The model under review builds one solid part; all positions refer to its coordinate system, in mm. A direction names the side the tool comes from. Round coordinates to 2 decimals unless told otherwise and drop trailing zeros. Loops run counter-clockwise (first coordinate to the right, second up) from the corner with the lowest first, then second, coordinate; pieces in that order, holes last. Notation, with made-up numbers: M 69.5,-17 L 89.5,-17 A28 ccw 89.5,10 Z; hole C -28,-16 d6. An arc over 180 degrees is marked long. One line per question, with ' | ' between items.
from build123d import *

# Parameters (mm, degrees)
CROQUIS1_W              = 40
CROQUIS1_H              = 41.5
CROQUIS1_R              = 2.5
SALIENTE_EXTRUIR1_DEPTH = 3
CROQUIS2_W              = 4
CROQUIS2_H              = 41.5
SALIENTE_EXTRUIR2_DEPTH = 45
CORTAR_EXTRUIR1_START   = 44
CROQUIS3_R              = 12.5
CROQUIS3_R_2            = 2.25
CORTAR_EXTRUIR1_DEPTH   = 4
SALIENTE_EXTRUIR4_START = 40
SALIENTE_EXTRUIR4_DEPTH = 4
CROQUIS6_W              = 40
CROQUIS6_H              = 9.5
CROQUIS6_H_2            = 9
SALIENTE_EXTRUIR5_DEPTH = 3
SALIENTE_EXTRUIR6_START = 46
CROQUIS7_W              = 40
CROQUIS7_H              = 61.549056497
CROQUIS7_R              = 2
SALIENTE_EXTRUIR6_DEPTH = 4


with BuildPart() as part:
    # Croquis1 → Saliente-Extruir1 (new body)
    with BuildSketch(Plane(origin=(0, 0, 0), x_dir=(1, 0, 0), z_dir=(0, 1, 0))):
        with Locations((20, -0.25)):
            Rectangle(CROQUIS1_W, CROQUIS1_H)
        with Locations((33.75, 14.25)):
            Circle(CROQUIS1_R, mode=Mode.SUBTRACT)
        with Locations((33.75, -14.75)):
            Circle(CROQUIS1_R, mode=Mode.SUBTRACT)
    extrude(amount=SALIENTE_EXTRUIR1_DEPTH)

    # Croquis2 → Saliente-Extruir2 (add)
    with BuildSketch(Plane(origin=(0, 0, 0), x_dir=(1, 0, 0), z_dir=(0, 1, 0))):
        with Locations((42, -0.25)):
            Rectangle(CROQUIS2_W, CROQUIS2_H)
    extrude(amount=SALIENTE_EXTRUIR2_DEPTH)

    # Croquis3 → Cortar-Extruir1 (cut)
    with BuildSketch(Plane(origin=(0, 0, 0), x_dir=(0, 0, -1), z_dir=(1, 0, 0)).offset(CORTAR_EXTRUIR1_START)):
        with Locations((-0.25, 24)):
            Circle(CROQUIS3_R)
        with Locations((15, 40)):
            Circle(CROQUIS3_R_2)
        with Locations((-15.5, 40)):
            Circle(CROQUIS3_R_2)
        with Locations((-15.5, 8)):
            Circle(CROQUIS3_R_2)
        with Locations((15, 8)):
            Circle(CROQUIS3_R_2)
    extrude(amount=-CORTAR_EXTRUIR1_DEPTH, mode=Mode.SUBTRACT)

    # Croquis5 → Saliente-Extruir4 (add)
    with BuildSketch(Plane(origin=(0, 0, 0), x_dir=(0, 0, -1), z_dir=(1, 0, 0)).offset(SALIENTE_EXTRUIR4_START)):
        Polygon((-21, 0), (-31, 0), (-31, 46), (30.549056497, 46), (30.5, 2.6158e-05), (20.5, 2.6158e-05), (20.5, 45), (-21, 45), align=None)
    extrude(amount=SALIENTE_EXTRUIR4_DEPTH)

    # Croquis6 → Saliente-Extruir5 (add)
    with BuildSketch(Plane(origin=(0, 0, 0), x_dir=(1, 0, 0), z_dir=(0, 1, 0))):
        with Locations((20, 25.25)):
            Rectangle(CROQUIS6_W, CROQUIS6_H)
        with Locations((20, -25.5)):
            Rectangle(CROQUIS6_W, CROQUIS6_H_2)
    extrude(amount=SALIENTE_EXTRUIR5_DEPTH)

    # Croquis7 → Saliente-Extruir6 (add)
    with BuildSketch(Plane(origin=(0, 0, 0), x_dir=(1, 0, 0), z_dir=(0, 1, 0)).offset(SALIENTE_EXTRUIR6_START)):
        with Locations((24, -0.225471752)):
            Rectangle(CROQUIS7_W, CROQUIS7_H)
        with Locations((34, 26.549056497)):
            Circle(CROQUIS7_R, mode=Mode.SUBTRACT)
        with Locations((34, -27)):
            Circle(CROQUIS7_R, mode=Mode.SUBTRACT)
    extrude(amount=SALIENTE_EXTRUIR6_DEPTH)


solid = part.part
1) Add section B-B on y = 24. State the section outline as (x, z) points.
Output values:
outline: M 40,-30.53 L 44,-30.53 L 44,-12.25 L 40,-12.25 Z; M 40,12.75 L 44,12.75 L 44,31 L 40,31 Z
2) Add section C-C on z = -15. State the section outline as (x, y) points, then the cut area to 3 significant figures.
Output values:
outline: M 0,0 L 31.37,0 L 31.37,3 L 0,3 Z; M 4,46 L 40,46 L 40,42.25 L 44,42.25 L 44,50 L 4,50 Z; M 36.13,0 L 44,0 L 44,5.75 L 40,5.75 L 40,3 L 36.13,3 Z; M 40,10.25 L 44,10.25 L 44,37.75 L 40,37.75 Z | area: 414 mm²
3) For line 1 (Z direction, x = 34, y = 49); line 2 (Y direction, x = 41.65, z = 15.5); line 3 (Z direction, x = 33.75, y = 1.45), list the stretches that pass through material, from the lowest coordinate up.
Output values:
line 1: z = -30.55 to -28.55, -24.55 to 25, 29 to 31 | line 2: y = 0 to 5.75, 10.25 to 37.75, 42.25 to 50 | line 3: z = -30 to -16.75, -11.75 to 12.25, 17.25 to 30
4) Mouldability with a two-part tool opening along Z and no side actions: class faces 5 (the flat face through (20, 1, -30)), 6 (the flat face through (42, 0, -26)), 7 (the cylindrical face through (42.028, 11.797, 2.96)) as +Z half, -Z half, draft (parallel to the pull), parting line (faces both ways), or undercut.
Output values:
face 5: -Z half | face 6: draft | face 7: undercut
5) Add section D-D on y = 40. State the section outline as (x, z) points, then the cut area to 3 significant figures.
Output values:
outline: M 40,-30.54 L 44,-30.54 L 44,-17.25 L 40,-17.25 Z; M 40,-12.75 L 44,-12.75 L 44,13.25 L 40,13.25 Z; M 40,17.75 L 44,17.75 L 44,31 L 40,31 Z | area: 210 mm²
6) Insertion check: P1, Ø2.5, axis at y = 8, z = -15, coming from the +X side; P2, Ø1, axis at x = 34.5, z = 13.5, coming from the -Y side; P3, Ø3.5, axis at x = 11, y = 1.5, coming from the +Z side; P4, Ø2.5, axis at x = 34, z = 27, coming from the +Y side. Each pin has a flat end and moves straight along its axis. Give the tip position at first contact, or say it passes through.
Output values:
P1: passes through | P2: stops at y = 46 | P3: stops at z = 30 | P4: stops at y = 3
7) Add section A-A on z = 0.25. State the section outline as (x, y) points, then the cut area to 3 significant figures.
Output values:
outline: M 0,0 L 44,0 L 44,11.5 L 40,11.5 L 40,3 L 0,3 Z; M 4,46 L 40,46 L 40,36.5 L 44,36.5 L 44,50 L 4,50 Z | area: 364 mm²
8) Machinability: for faces 1 (the flat face through (20, 1, 30)), 2 (the cylindrical face through (34.923, 47.972, -24.775)), 3 (the flat face through (4, 48, 1)), 4 (the cylindrical face through (33.21, 1.48, 17.19)), which of the approach directions +Z, -Z, +X, -X, +Y, -Y give a long, thin tool a straight path to every point of the face, cutting with its end or side? Answer none if there is none.
Output values:
face 1: +Z, -X, -Y | face 2: +Y | face 3: +Z, -Z, -X, +Y | face 4: -Y
